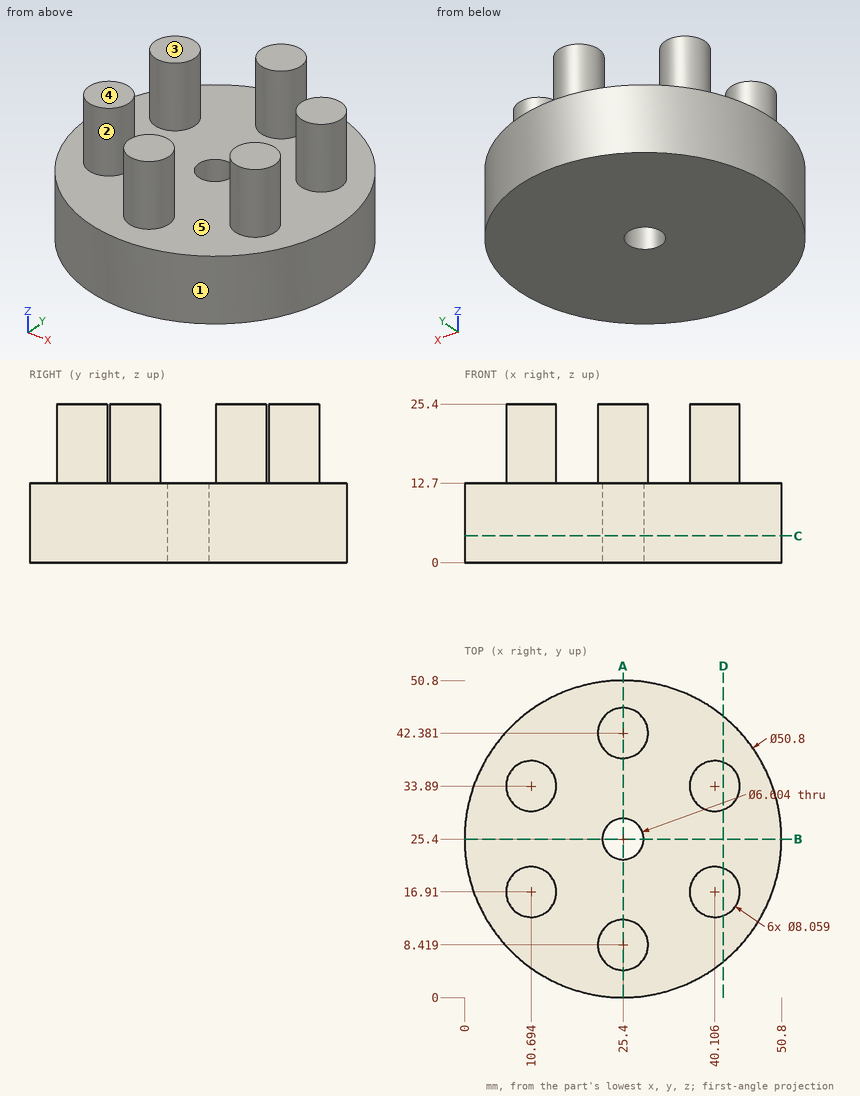
The figure shows three views and two pictorial views of one solid part (mm, origin at its lowest corner). Answer the questions. A direction names the side the tool comes from. Coordinates: 2 decimals unless noted, no trailing zeros. Loops run counter-clockwise (first coordinate to the right, second up) from the corner with the lowest first, then second, coordinate; pieces in that order, holes last. Notation, with made-up numbers: (-31, -29) -> (13, -29) arc R12 ccw to (13, -15) -> close; hole circle Ø10 at (-2, 67). An arc over 180 degrees is marked (long way). Write item = value, one per line. Start each with the question number.
1) A cutting plane is placed at C-C (z = 4.25). Give the vertices of the cut face in (x, y).
2) The mould has two halves that part along X. Classify the marked faces 1, 2 and 3: released by +X, released by -X, zero draft, split by the parting line, or undercut.
3) A cutting plane is placed at D-D (x = 41.5). Give the vertices of the cut face in (y, z) (1 decimal), then the cut area to 3 significant figures.
4) A cutting plane is placed at B-B (y = 25.4). Give the vertices of the cut face in (x, z).
5) A tool of negligible diameter and unlimited length cuts with its end or side. For the marked faces 4 and 5, from which of +Z, -Z, +X, -X, +Y, -Y can it reach the whole face along a straight path? Write none if from no direction.
6) Straight lines are drawn through the part: line 1 (Y direction, x = 25.4, z = 7.75); line 2 (Z direction, x = 47.5, y = 27); line 3 (Y direction, x = 7, z = 21.25) (1 decimal). For each, find the intervals that lie inside material, in ascending order. Write a range as from..to.
7) Given pin 1 Ø1.5 at (x, z) = (37.5, 18) entering from -Y; pin 2 Ø5 at (x, z) = (40.5, 4.5) entering from -Y (1 decimal); pin 3 Ø5 at (y, z) = (39, 19) entering from +X (1 decimal); pin 4 Ø1 at (x, z) = (35.5, 22.5) entering from +Y, each flat-ended and moving along its own axis, determine where each tip first touches the part or whether it passes through.
8) A cutting plane is placed at A-A (x = 25.4). Give the vertices of the cut face in (y, z), then the cut area to 3 significant figures.
Responses:
q1.outline = circle Ø50.8 at (25.4, 25.4); hole circle Ø6.6 at (25.4, 25.4)
q2.face_1 = split by the parting line
q2.face_2 = undercut
q2.face_3 = zero draft
q3.outline = (5.8, 0) -> (45, 0) -> (45, 12.7) -> (37.7, 12.7) -> (37.7, 25.4) -> (30.1, 25.4) -> (30.1, 12.7) -> (20.7, 12.7) -> (20.7, 25.4) -> (13.1, 25.4) -> (13.1, 12.7) -> (5.8, 12.7) -> close
q3.area = 691 mm²
q4.outline = (0, 0) -> (22.1, 0) -> (22.1, 12.7) -> (0, 12.7) -> close; (28.7, 0) -> (50.8, 0) -> (50.8, 12.7) -> (28.7, 12.7) -> close
q5.face_4 = +Z, +X, -X, +Y, -Y
q5.face_5 = +Z
q6.line_1 = 0..22.1, 28.7..50.8
q6.line_2 = 0..12.7
q6.line_3 = 15.3..18.5, 32.3..35.5
q7.pin_1 = 13.33
q7.pin_2 = 3.3
q7.pin_3 = 43.2
q7.pin_4 = through
q8.outline = (0, 0) -> (22.1, 0) -> (22.1, 12.7) -> (12.45, 12.7) -> (12.45, 25.4) -> (4.39, 25.4) -> (4.39, 12.7) -> (0, 12.7) -> close; (28.7, 0) -> (50.8, 0) -> (50.8, 12.7) -> (46.41, 12.7) -> (46.41, 25.4) -> (38.35, 25.4) -> (38.35, 12.7) -> (28.7, 12.7) -> close
q8.area = 766 mm²
